Autodesk Inventor part; units mm, degrees
ref_plane "Work Plane1" through (-6.8079, 0, 0) normal (0, 0, -1) x (1, 0, 0)
ref_plane "YZ Plane" through (0, 0, 0) normal (1, 0, 0) x (0, 1, 0)
ref_plane "XZ Plane" through (0, 0, 0) normal (0, 1, 0) x (-1, 0, 0)
sketch "Sketch1" plane through (0, 0, 0) normal (1, 0, 0) x (0, 1, 0)
  line L0 (1.5877, -2.75) -> (-1.5877, -2.75)
  line L1 (-1.5877, -2.75) -> (-3.1754, 0)
  line L2 (-3.1754, 0) -> (-1.5877, 2.75)
  line L3 (-1.5877, 2.75) -> (1.5877, 2.75)
  line L4 (1.5877, 2.75) -> (3.1754, 0)
  line L5 (3.1754, 0) -> (1.5877, -2.75)
  point P0 (0, 0)
  point P1 (0, 0)
  dimension "d0" = 6.3509
extrude "Body" add sketch "Sketch1" along normal blind 1.78
sketch "Sketch2" plane through (1.78, 0, 0) normal (1, 0, 0) x (0, 0, -1)
  point P0 (0, 0)
hole "Thread" at (1.78, 0, 0) direction (-1, 0, 0) diameter 2.459 end through all
chamfer "Chamfer2" distance 0.2706 angle 30 1 edges at (1.78, 0, 1.2295) measured on face at (1.78, -1.925, 1.1495)
chamfer "Chamfer1" distance 0.2706 angle 30 1 edges at (0, 0, 1.2295) measured on face at (0, -1.925, 1.1495)
ref_plane "Work Plane1" through (-6.8079, 0, 0) normal (0, 0, -1) x (1, 0, 0)
equation "\"d0\" = 1.1547 * SW"
equation "\"d1\" = KOH"
equation "\"d12\" = -0.5 * GD1 + 0.5 * NND"
equation "\"d19\" = -0.5 * GD1 + 0.5 * NND"
equation "\"d10\" = -0.5 * GD1 + 0.5 * NND"
equation "\"d18\" = -0.5 * GD1 + 0.5 * NND"
equation "\"NND\" = 3"
equation "\"KOH\" = 1.78"
equation "\"SW\" = 5.5"
equation "\"GUL\" = 0.541266 * PTC"
equation "\"THREADDIA\" = 3"
equation "\"TOA\" = 30deg"
equation "\"PTC\" = 0.5"
equation "\"E0\" = 1.155 * SW"
equation "\"GAL\" = 0.541266 * PTC"
properties part number "AS 1474 - M3" material "Steel, Mild"
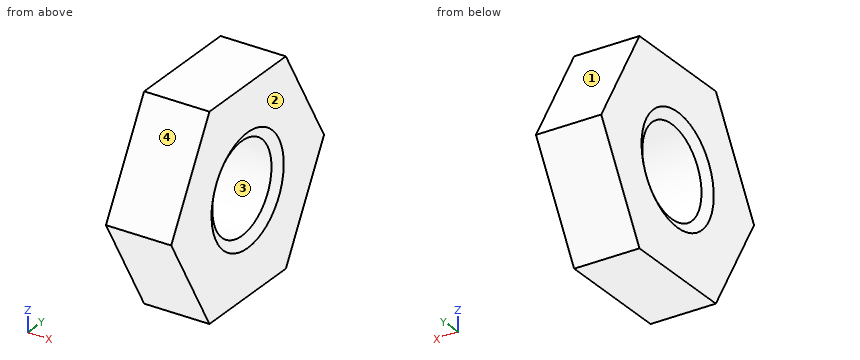
Source: CAD feature listing. Evaluate the final solid. Frame: model axes, mm. Face numbers are marked on the shaded views. Coordinates: 2 decimals unless noted, no trailing zeros. Order: outer loops, then holes, each group sorted by start corner. A loop starts at its lowest first (then second) coordinate and runs counter-clockwise, first axis right, second up. Notation, with made-up numbers: (-18.5, 9.25) - (-5.5, 9.25) arc R17 ccw to (-5.5, 42.25) - close; hole circle Ø3 at (-6, 54.5). An arc over 180 degrees is marked (long way). One line per item, written item: value.
1) Cut plane B-B on x = 0.4. Output: boundary loops of the cut face in (y, z), plus the area to 3 significant figures.
Computed values:
outline: (-3.18, 0) - (-1.59, -2.75) - (1.59, -2.75) - (3.18, 0) - (1.59, 2.75) - (-1.59, 2.75) - close; hole circle Ø2.46 at (0, 0)
area: 21.4 mm^2
2) Ray query, line 1 (Z direction, x = 0.9, y = 0); line 2 (Y direction, x = 0.6, z = -1); line 3 (Y direction, x = 1.35, z = -0.8). Return the intervals inside material, ascending. Write a range as [from, to].
Computed values:
line 1: z = [-2.75, -1.23], [1.23, 2.75]
line 2: y = [-2.6, -0.72], [0.72, 2.6]
line 3: y = [-2.71, -0.93], [0.93, 2.71]
3) Mould query, pull axis Y, two halves, no side actions, for the marked faces 1, 2, 3 and 4. Classes: released by +Y, released by -Y, zero draft, split by the parting line, or undercut.
Computed values:
face 1: released by +Y
face 2: zero draft
face 3: undercut
face 4: released by -Y
4) Cut plane C-C on y = -2. Output: boundary loops of the cut face in (x, z), plus the area to 3 significant figures.
Computed values:
outline: (0, -2.04) - (1.78, -2.04) - (1.78, 2.04) - (0, 2.04) - close
area: 7.25 mm^2
5) Cut plane A-A on y = 0. Output: boundary loops of the cut face in (x, z).
Computed values:
outline: (0, -2.75) - (1.78, -2.75) - (1.78, -1.5) - (1.62, -1.23) - (0.16, -1.23) - (0, -1.5) - close; (0, 1.5) - (0.16, 1.23) - (1.62, 1.23) - (1.78, 1.5) - (1.78, 2.75) - (0, 2.75) - close
6) Cut plane D-D on z = -1.85. Output: boundary loops of the cut face in (x, y).
Computed values:
outline: (0, -2.11) - (1.78, -2.11) - (1.78, 2.11) - (0, 2.11) - close
